from build123d import *

# Parameters (mm, degrees)
F1_DEPTH = 2.54


with BuildPart() as f1:
    # F0 (on Top) → F1 (new body)
    with BuildSketch(Plane.XY):
        with BuildLine():
            ThreePointArc((2.327948453, 1.016), (2.4864220348, 0.518946495), (2.54, 0))
            Line((2.54, 0), (4.572, 0))
            ThreePointArc((4.572, 0), (4.4755596627, 0.9341036909), (4.1903072155, 1.8288))
            Line((4.1903072155, 1.8288), (2.327948453, 1.016))
        make_face()
        with BuildLine():
            Line((4.572, 0), (2.54, 0))
            ThreePointArc((2.54, 0), (2.1251164674, -1.3912152961), (1.016, -2.327948453))
            Line((1.016, -2.327948453), (1.8288, -4.1903072155))
            ThreePointArc((1.8288, -4.1903072155), (3.8252096413, -2.5041875329), (4.572, 0))
        make_face()
        with BuildLine():
            ThreePointArc((-2.327948453, 1.016), (0, 2.54), (2.327948453, 1.016))
            Line((2.327948453, 1.016), (4.1903072155, 1.8288))
            ThreePointArc((4.1903072155, 1.8288), (0, 4.572), (-4.1903072155, 1.8288))
            Line((-4.1903072155, 1.8288), (-2.327948453, 1.016))
        make_face()
        with BuildLine():
            ThreePointArc((-2.54, 0), (-2.4864220348, 0.518946495), (-2.327948453, 1.016))
            Line((-2.327948453, 1.016), (-4.1903072155, 1.8288))
            ThreePointArc((-4.1903072155, 1.8288), (-4.4755596627, 0.9341036909), (-4.572, 0))
            Line((-4.572, 0), (-2.54, 0))
        make_face()
        with BuildLine():
            Line((0.9144, -4.4796268416), (0.508, -2.4886815787))
            ThreePointArc((0.508, -2.4886815787), (-1.6064370514, -1.9674755399), (-2.54, 0))
            Line((-2.54, 0), (-4.572, 0))
            ThreePointArc((-4.572, 0), (-2.8915866925, -3.5414559718), (0.9144, -4.4796268416))
        make_face()
        with BuildLine():
            ThreePointArc((1.016, -2.327948453), (0.7662263272, -2.4216724005), (0.508, -2.4886815787))
            Line((0.508, -2.4886815787), (0.9144, -4.4796268416))
            ThreePointArc((0.9144, -4.4796268416), (1.3792073889, -4.359010321), (1.8288, -4.1903072155))
            Line((1.8288, -4.1903072155), (1.016, -2.327948453))
        make_face()
        with BuildLine():
            ThreePointArc((4.1903072155, 1.8288), (4.4755596627, 0.9341036909), (4.572, 0))
            Line((4.572, 0), (7.62, 0))
            ThreePointArc((7.62, 0), (7.4592661045, 1.5568394849), (6.9838453591, 3.048))
            Line((6.9838453591, 3.048), (4.1903072155, 1.8288))
        make_face()
        with BuildLine():
            ThreePointArc((-4.1903072155, 1.8288), (0, 4.572), (4.1903072155, 1.8288))
            Line((4.1903072155, 1.8288), (6.9838453591, 3.048))
            ThreePointArc((6.9838453591, 3.048), (0, 7.62), (-6.9838453591, 3.048))
            Line((-6.9838453591, 3.048), (-4.1903072155, 1.8288))
        make_face()
        with BuildLine():
            ThreePointArc((-4.572, 0), (-4.4755596627, 0.9341036909), (-4.1903072155, 1.8288))
            Line((-4.1903072155, 1.8288), (-6.9838453591, 3.048))
            ThreePointArc((-6.9838453591, 3.048), (-7.4592661045, 1.5568394849), (-7.62, 0))
            Line((-7.62, 0), (-4.572, 0))
        make_face()
        with BuildLine():
            ThreePointArc((1.8288, -4.1903072155), (1.3792073889, -4.359010321), (0.9144, -4.4796268416))
            Line((0.9144, -4.4796268416), (1.524, -7.466044736))
            ThreePointArc((1.524, -7.466044736), (2.2986789815, -7.2650172016), (3.048, -6.9838453591))
            Line((3.048, -6.9838453591), (1.8288, -4.1903072155))
        make_face()
        with BuildLine():
            ThreePointArc((-6.9838453591, 3.048), (0, 7.62), (6.9838453591, 3.048))
            Line((6.9838453591, 3.048), (11.6397422652, 5.08))
            ThreePointArc((11.6397422652, 5.08), (0, 12.7), (-11.6397422652, 5.08))
            Line((-11.6397422652, 5.08), (-6.9838453591, 3.048))
        make_face()
        with BuildLine():
            ThreePointArc((3.048, -6.9838453591), (2.2986789815, -7.2650172016), (1.524, -7.466044736))
            Line((1.524, -7.466044736), (2.54, -12.4434078933))
            ThreePointArc((2.54, -12.4434078933), (3.8311316358, -12.1083620027), (5.08, -11.6397422652))
            Line((5.08, -11.6397422652), (3.048, -6.9838453591))
        make_face()
    extrude(amount=F1_DEPTH)


solid = f1.part
Here's how the part is built. I have some questions about the finished solid (model axes, mm). A direction names the side the tool comes from. Give positions to 0.01 mm unless a question says otherwise; leave off trailing zeros. Order: outer loops, then holes, each group sorted by start corner. A loop starts at its lowest first (then second) coordinate and runs counter-clockwise, first axis right, second up. Notation, with made-up numbers: M -39.75,9 L -22.75,9 A22 cw -22.75,37 Z; hole C -0.75,-2 d7. An arc over 180 degrees is marked long. Answer as a JSON object with one key per item and string values. Group by question number.
1) Suppose I cut it at A-A, the plane z = 1.55. Write out the boundary of the cut face in (x, y).
2) Suppose I cut it at B-B, the plane x = -1. Write out the boundary of the cut face in (y, z).
3) We'd pull the mould along Y, two halves only. Please class faces 4 (the flat face through (0, 6, 0)), 5 (the cylindrical face through (-7.455, 1.578, 1.252)), 6 (the cylindrical face through (0.2, 12.7, 1.3)): pulls with the +Y half, pulls with the -Y half, needs draft (parallel to the pull), parting line crosses it, or undercut.
4) Suppose I cut it at C-C, the plane y = 8.25. Write out the boundary of the cut face in (x, z), plus the area to 3 significant figures.
5) I'm going to push flat-ended pins straight in: pin 1 Ø4 at (x, y) = (6, -3) entering from -Z; pin 2 Ø1.3 at (x, z) = (5.5, 2) entering from -Y; pin 3 Ø0.8 at (x, z) = (-7, 1) entering from -Y. Where does each tip first touch, or does it pass through?
6) Suppose I cut it at D-D, the plane x = 8. Write out the boundary of the cut face in (y, z), plus the area to 3 significant figures.
7) On a 3-axis mill with a long thin cutter (end or side, diameter ignored), from which of +Z, -Z, +X, -X, +Y, -Y can I reach the whole of each face in a straight line? I mean faces 1 (the flat face through (6, 0, 1)), 2 (the cylindrical face through (3.813, -12.114, 1.252)), 3 (the flat face through (-6, 0, 1)). Say none if no direction works.
8) Please list where these lines run through material, in increasing order: L1, parallel to Y at x = -0.25, z = 1.15; L2, parallel to Y at x = -6, z = 1.4; L3, parallel to Y at x = 0.5, z = 1.4. Write a range as [from, to].
Results found:
{
 "1": {"outline": "M -11.64,5.08 L -6.98,3.05 A7.62 ccw -7.62,0 L -4.57,0 A4.57 ccw 0.91,-4.48 L 2.54,-12.44 A12.7 ccw 5.08,-11.64 L 1.83,-4.19 A4.57 ccw 4.57,0 L 7.62,0 A7.62 ccw 6.98,3.05 L 11.64,5.08 A12.7 ccw Z; hole C 0,0 d5.08"},
 "2": {"outline": "M -4.46,0 L -2.33,0 L -2.33,2.54 L -4.46,2.54 Z; M 2.33,0 L 12.66,0 L 12.66,2.54 L 2.33,2.54 Z"},
 "3": {"face 4": "needs draft", "face 5": "undercut", "face 6": "pulls with the +Y half"},
 "4": {"outline": "M -9.66,0 L 9.66,0 L 9.66,2.54 L -9.66,2.54 Z", "area": "49.0 mm²"},
 "5": {"pin 1": "through", "pin 2": "y = -11.74", "pin 3": "y = 0"},
 "6": {"outline": "M 3.49,0 L 9.86,0 L 9.86,2.54 L 3.49,2.54 Z", "area": "16.2 mm²"},
 "7": {"face 1": "+Z, -Z, +X", "face 2": "+Z, -Z, +X, -Y", "face 3": "+Z, -Z, -X, -Y"},
 "8": {"L1": "[-4.57, -2.53], [2.53, 12.7]", "L2": "[0, 11.19]", "L3": "[-4.54, -2.49], [2.49, 12.69]"}
}
